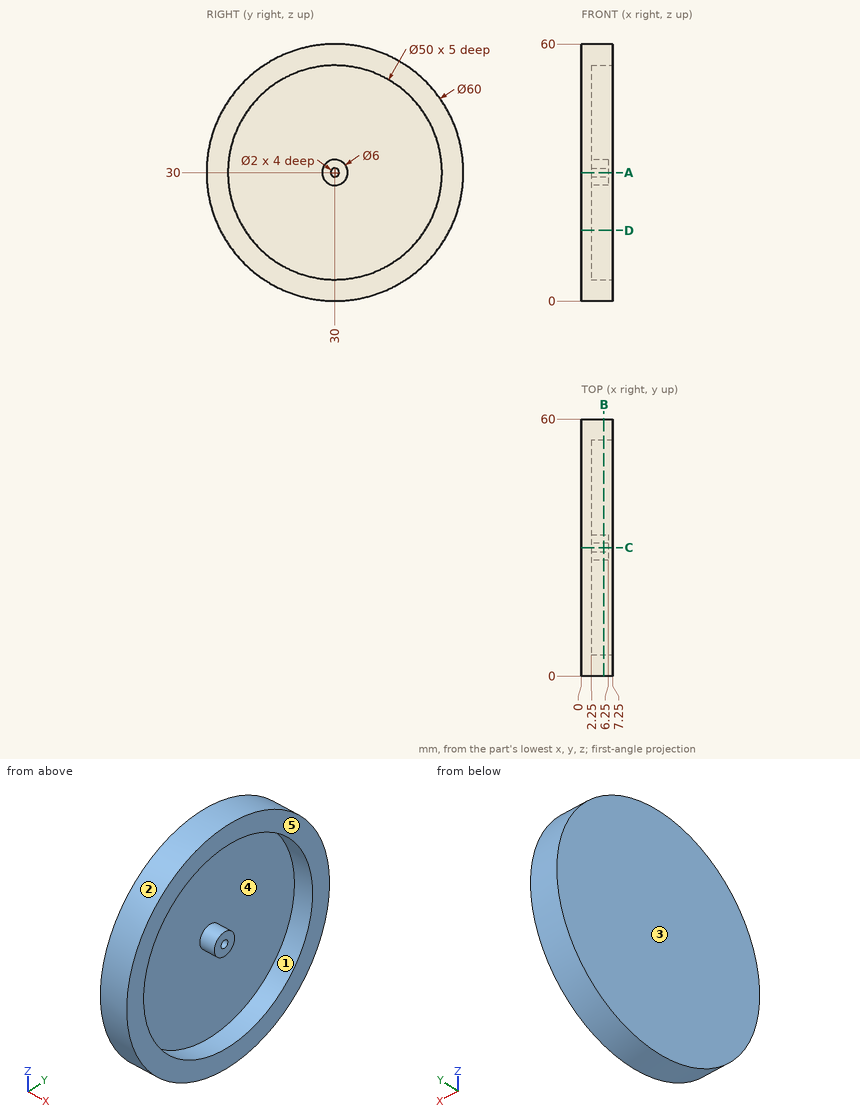
Answer from the drawing. Dimensions are ordinates in mm from the lowest x, y and z of the part. A direction names the side the tool comes from. Round coordinates to 2 decimals unless told otherwise and drop trailing zeros. Loops run counter-clockwise (first coordinate to the right, second up) from the corner with the lowest first, then second, coordinate; pieces in that order, holes last.
Q1. Consider probe 1 along Z at (x, y) = (3.5, 30); probe 2 along X at (y, z) = (23.5, 49); probe 3 along Z at (x, y) = (4, 41.5). Determine where each line is inside the solid, lowest interval first.
Q2. Which of the six approach directions +Z, -Z, +X, -X, +Y, -Y give full straight-line access (tool end or side, diameter ignored) to the marked faces 4 and 5?
Q3. Section B-B on x = 5.25 is taken. Write down the section's boundary in (y, z), and give its area (3 significant figures).
Q4. Section A-A on z = 30 is taken. Write down the section's boundary in (x, y), and give its area (3 significant figures).
Q5. Each of these flat-tipped pins is pushed along its axis until it touches: pin 1 (4 mm diameter, centred on x = 5, y = 38.5, fed in from +Z); pin 2 (25 mm diameter, centred on y = 31, z = 30, fed in from +X); pin 3 (1.8 mm diameter, centred on y = 30, z = 30, fed in from +X). Where does it stop, or does it pass through?
Q6. Determine the mould class of the marked faces 1, 2 and 3 for opening direction Z: released by +Z, released by -Z, zero draft, split by the parting line, or undercut.
Q7. Section D-D on z = 16.5 is taken. Write down the section's boundary in (x, y).
Output:
1. probe 1: z = 0 to 5, 27 to 29, 31 to 33, 55 to 60
1. probe 2: x = 0 to 2.25
1. probe 3: z = 2.29 to 7.8, 52.2 to 57.71
2. face 4: +X
2. face 5: +Z, -Z, +X, +Y, -Y
3. outline: circle Ø60 at (30, 30); circle Ø6 at (30, 30); hole circle Ø50 at (30, 30); hole circle Ø2 at (30, 30)
3. area: 889 mm2
4. outline: (0, 0) - (7.25, 0) - (7.25, 5) - (2.25, 5) - (2.25, 27) - (6.25, 27) - (6.25, 29) - (2.25, 29) - (2.25, 31) - (6.25, 31) - (6.25, 33) - (2.25, 33) - (2.25, 55) - (7.25, 55) - (7.25, 60) - (0, 60) - close
4. area: 201 mm2
5. pin 1: stops at z = 59.29
5. pin 2: stops at x = 6.25
5. pin 3: stops at x = 2.25
6. face 1: undercut
6. face 2: split by the parting line
6. face 3: zero draft
7. outline: (0, 3.21) - (7.25, 3.21) - (7.25, 8.96) - (2.25, 8.96) - (2.25, 51.04) - (7.25, 51.04) - (7.25, 56.79) - (0, 56.79) - close
